Verification items for the finished model (mm, model axes). Give positions to 0.01 mm unless a question says otherwise; leave off trailing zeros. Order: outer loops, then holes, each group sorted by start corner. A loop starts at its lowest first (then second) coordinate and runs counter-clockwise, first axis right, second up.
(1) Sectioned sample at C-C on y = -9.5. Record the cut outline in (x, z), plus the area to 4 significant figures.
(2) Sectioned sample at A-A on z = 269. Record the cut outline in (x, y).
(3) Scan lines: L1, parallel to Y at x = -16.85, z = 235; L2, parallel to X at y = -14.55, z = 316.5; L3, parallel to Y at x = -1.5, z = 275.5. Record each from-to range of solid material in increasing order.
(4) Gauge pin test, flat ends, axial feed: pin 1 (10 mm diameter, centred on x = -0.5, z = 274.5, fed in from +Y); pin 2 (2.5 mm diameter, centred on x = -7.43, z = 90, fed in from +Y); pin 3 (4 mm diameter, centred on y = -5.23, z = 316.5, fed in from +X). Record the tip position at first contact, or that the pin passes through.
(5) Sectioned sample at B-B on x = -12.5. Record the cut outline in (y, z), plus the area to 4 significant figures.
```python
from build123d import *

# Parameters (mm, degrees)
EXTRUSION1_DEPTH = 325
ESQUISSE2_R      = 1.5
EXTRUSION2_DEPTH = 300
ESQUISSE3_R      = 1.5
EXTRUSION3_DEPTH = 300


with BuildPart() as part:
    # Esquisse1 → Extrusion1 (new body)
    with BuildSketch(Plane.XY):
        Polygon((-17.43168638, 4.773368421), (-17.43168638, -15.226631579), (2.56831362, -15.226631579), (2.56831362, -13.726631579), (-15.93168638, -13.726631579), (-15.93168638, 4.773368421), align=None)
    extrude(amount=EXTRUSION1_DEPTH)

    # Esquisse2 → Extrusion2 (cut)
    with BuildSketch(Plane(origin=(0, -13.726631579, 0), x_dir=(-1, 0, 0), z_dir=(0, 1, 0))):
        with Locations((7.43168638, 8.5)):
            Circle(ESQUISSE2_R)
        with Locations((7.43168638, 316.5)):
            Circle(ESQUISSE2_R)
        with Locations((7.43168638, 235)):
            Circle(ESQUISSE2_R)
        with Locations((7.43168638, 90)):
            Circle(ESQUISSE2_R)
    extrude(amount=-EXTRUSION2_DEPTH, mode=Mode.SUBTRACT)

    # Esquisse3 → Extrusion3 (cut)
    with BuildSketch(Plane(origin=(-15.93168638, 0, 0), x_dir=(0, 0, -1), z_dir=(1, 0, 0))):
        with Locations((-316.5, -5.226631579)):
            Circle(ESQUISSE3_R)
        with Locations((-8.5, -5.226631579)):
            Circle(ESQUISSE3_R)
        with Locations((-235, -5.226631579)):
            Circle(ESQUISSE3_R)
        with Locations((-90, -5.226631579)):
            Circle(ESQUISSE3_R)
        with Locations((-113, -3.726631579)):
            Circle(ESQUISSE3_R)
        with Locations((-156, -3.726631579)):
            Circle(ESQUISSE3_R)
    extrude(amount=-EXTRUSION3_DEPTH, mode=Mode.SUBTRACT)


solid = part.part
```
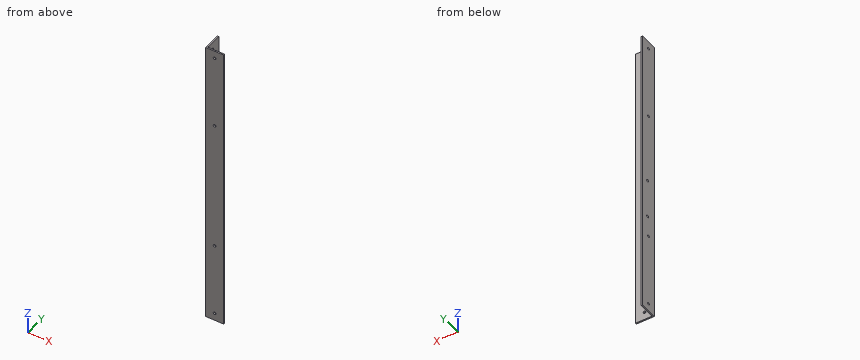
Ans:
1. outline: (-17.43, 0) - (-15.93, 0) - (-15.93, 325) - (-17.43, 325) - close
1. area: 487.5 mm2
2. outline: (-17.43, -15.23) - (2.57, -15.23) - (2.57, -13.73) - (-15.93, -13.73) - (-15.93, 4.77) - (-17.43, 4.77) - close
3. L1: y = -15.23 to -6.73, -3.73 to 4.77
3. L2: x = -17.43 to -8.93, -5.93 to 2.57
3. L3: y = -15.23 to -13.73
4. pin 1: stops at y = -13.73
4. pin 2: passes through
4. pin 3: stops at x = -15.93
5. outline: (-15.23, 0) - (-13.73, 0) - (-13.73, 325) - (-15.23, 325) - close
5. area: 487.5 mm2
